Job drawing, mm, ordinate dimensions from the low corner. One solid piece. Round coordinates to 2 decimals unless told otherwise and drop trailing zeros. Order: outer loops, then holes, each group sorted by start corner. A loop starts at its lowest first (then second) coordinate and runs counter-clockwise, first axis right, second up. Notation, with made-up numbers: (51.25, -10.5) -> (82.25, -10.5) arc R23 cw to (82.25, 3.5) -> close; hole circle Ø8 at (-20, 84.25). An arc over 180 degrees is marked (long way). Write item = value, one per line.
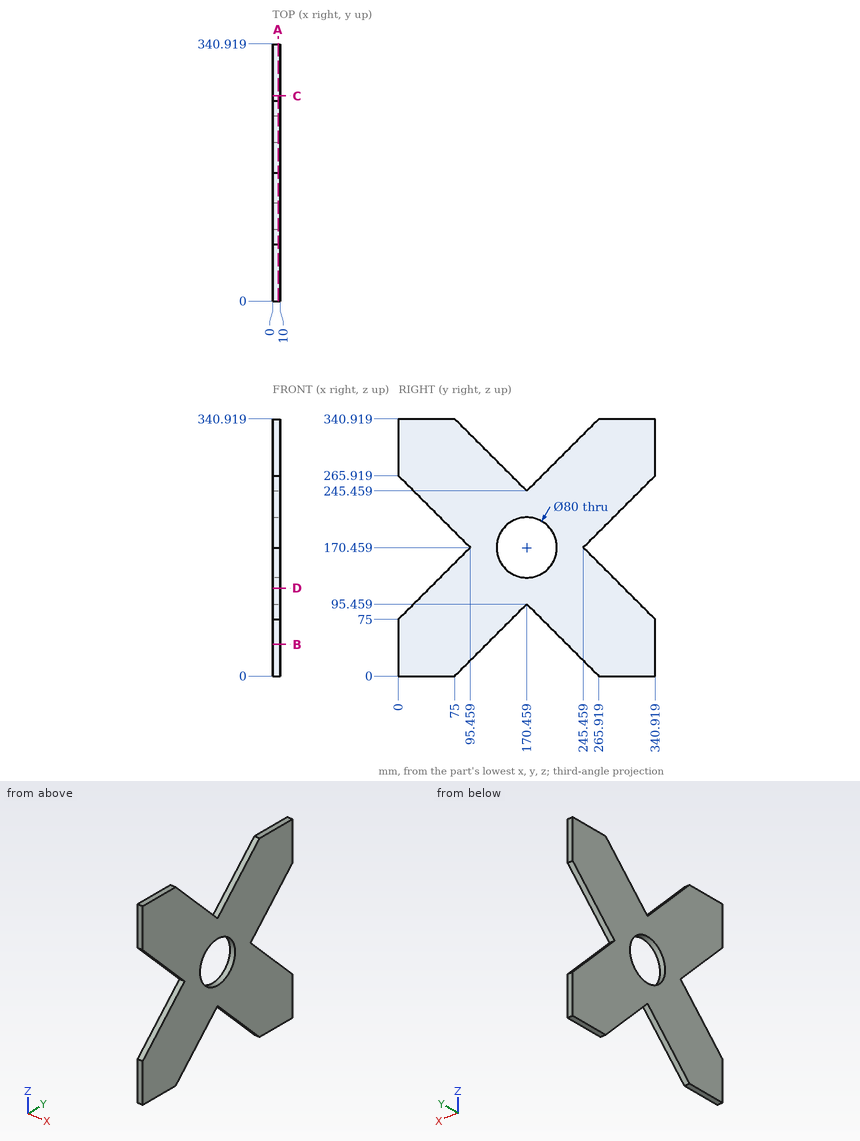
Q1. Cut at B-B, the plane z = 42. List the corners of the cut face in (x, y), and give its area (3 significant figures).
Check values:
outline = (0, 0) -> (10, 0) -> (10, 117) -> (0, 117) -> close; (0, 223.92) -> (10, 223.92) -> (10, 340.92) -> (0, 340.92) -> close
area = 2,340 mm²
Q2. Probe probe 1 along Y at (x, z) = (4, 280.5); probe 2 along Z at (x, y) = (3.5, 42.5); probe 3 along Z at (x, y) = (3.5, 250.5). List the from-to ranges inside material, lowest first.
Check values:
probe_1 = 0 to 135.42, 205.5 to 340.92
probe_2 = 0 to 117.5, 223.42 to 340.92
probe_3 = 15.42 to 165.42, 175.5 to 325.5
Q3. Cut at D-D, the plane z = 116.5. List the corners of the cut face in (x, y).
Check values:
outline = (0, 41.5) -> (10, 41.5) -> (10, 299.42) -> (0, 299.42) -> close
Q4. Cut at C-C, the plane y = 272. List the corners of the cut face in (x, z).
Check values:
outline = (0, 0) -> (10, 0) -> (10, 143.92) -> (0, 143.92) -> close; (0, 197) -> (10, 197) -> (10, 340.92) -> (0, 340.92) -> close
Q5. Flat gauge pins, fed straight in: pin 1 (2 mm diameter, centred on x = 2.5, y = 216.5, fed in from -Z); pin 2 (2 mm diameter, centred on x = 2, z = 203.5, fed in from +Y); pin 3 (1.5 mm diameter, centred on x = 2, y = 215, fed in from +Z). Where does each tip first touch, or does it go through?
Check values:
pin_1 = 48.42
pin_2 = 279.5
pin_3 = 290.75
Q6. Cut at A-A, the plane x = 7. List the corners of the cut face in (y, z), and give its area (4 significant figures).
Check values:
outline = (0, 0) -> (75, 0) -> (170.46, 95.46) -> (265.92, 0) -> (340.92, 0) -> (340.92, 75) -> (245.46, 170.46) -> (340.92, 265.92) -> (340.92, 340.92) -> (265.92, 340.92) -> (170.46, 245.46) -> (75, 340.92) -> (0, 340.92) -> (0, 265.92) -> (95.46, 170.46) -> (0, 75) -> close; hole circle Ø80 at (170.46, 170.46)
area = 74,750 mm²
